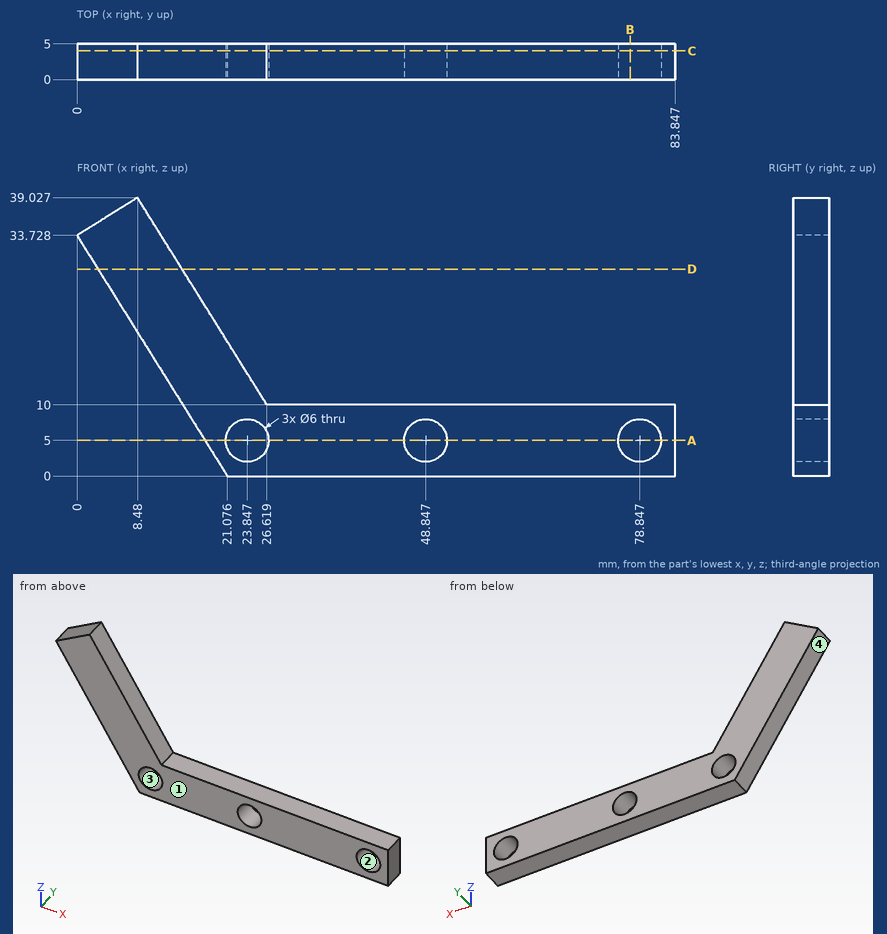
Can you work these out from the drawing? Everything is in mm from the part's minimum corner. Round coordinates to 2 decimals unless told otherwise and drop trailing zeros. Loops run counter-clockwise (first coordinate to the right, second up) from the corner with the lowest first, then second, coordinate; pieces in that order, holes last. Notation, with made-up numbers: M 75,-29.5 L 110,-29.5 A19 cw 110,-20.5 Z; hole C 23,-39 d8. An arc over 180 degrees is marked long. Answer in a Markdown table with one row per item.
1. Please list where these lines run through material, in increasing order: line 1 (X direction, y = 1.95, z = 5); line 2 (X direction, y = 0.3, z = 7) (1 decimal); line 3 (Z direction, x = 45, y = 3.7). Write a range as from..to.
Established:
| item | result |
|---|---|
| line 1 | 17.95..20.85, 26.85..45.85, 51.85..75.85, 81.85..83.85 |
| line 2 | 16.7..21.6, 26.1..46.6, 51.1..76.6, 81.1..83.8 |
| line 3 | 0..10 |
2. Thinking about a two-plate mould opening in X: for the marked faces 1, 2, 3 and 4, which applies, pulls with the +X half, pulls with the -X half, needs draft (parallel to the pull), parting line crosses it, or undercut?
Established:
| item | result |
|---|---|
| face 1 | needs draft |
| face 2 | undercut |
| face 3 | undercut |
| face 4 | pulls with the -X half |
3. If we section it at A-A, the plane z = 5: Please give me the cut outline in (x, y).
Established:
| item | result |
|---|---|
| outline | M 17.95,0 L 20.85,0 L 20.85,5 L 17.95,5 Z; M 26.85,0 L 45.85,0 L 45.85,5 L 26.85,5 Z; M 51.85,0 L 75.85,0 L 75.85,5 L 51.85,5 Z; M 81.85,0 L 83.85,0 L 83.85,5 L 81.85,5 Z |
4. If we section it at D-D, the plane z = 29: Please give me the cut outline in (x, y) (1 decimal).
Established:
| item | result |
|---|---|
| outline | M 3,0 L 14.7,0 L 14.7,5 L 3,5 Z |
5. I'm going to push flat-ended pins straight in: pin 1 Ø10 at (x, z) = (13, 33.5) entering from +Y; pin 2 Ø2 at (y, z) = (4.5, 16.5) entering from -X; pin 3 Ø1.5 at (y, z) = (2.5, 24.5) entering from +X. Where does each tip first touch, or does it pass through?
Established:
| item | result |
|---|---|
| pin 1 | y = 5 |
| pin 2 | x = 10.14 |
| pin 3 | x = 18.03 |
6. If we section it at C-C, the plane y = 4.05: Please give me the cut outline in (x, z) (1 decimal).
Established:
| item | result |
|---|---|
| outline | M 0,33.7 L 21.1,0 L 83.8,0 L 83.8,10 L 26.6,10 L 8.5,39 Z; hole C 23.8,5 d6; hole C 48.8,5 d6; hole C 78.8,5 d6 |
7. If we section it at B-B, the plane x = 77.5: Please give me the cut outline in (y, z).
Established:
| item | result |
|---|---|
| outline | M 0,0 L 5,0 L 5,2.32 L 0,2.32 Z; M 0,7.68 L 5,7.68 L 5,10 L 0,10 Z |
